Design review of the part built by this model. Coordinates are the model's own, in mm. A direction names the side the tool comes from. Coordinates: 2 decimals unless noted, no trailing zeros. Write each loop counter-clockwise with the first axis right and the second up, starting at its lowest first coordinate (ties: lowest second). Pieces come first, ordered by that corner, then holes.
Q1. For L1, parallel to Z at x = -5.5, y = 0; L2, parallel to Z at x = -6, y = 1.25; L3, parallel to Y at x = 3.75, z = 69.5, list the stretches that pass through material, from the lowest coordinate up.
Q2. The part is to be moulded in two halves that separate along Z. For faces 4 (the flat face through (13.97, 0, 50)), 5 (the cylindrical face through (-5.211, 0.112, 63.515)), 6 (the flat face through (0, 0, 101.6)), say which applies: released by +Z, released by -Z, zero draft, split by the parting line, or undercut.
Q3. Take a section at B-B, the plane z = 70.5. Write out the cut boundary in (x, y), plus the area to 3 significant figures.
Q4. Take a section at A-A, the plane y = 0. Write out the cut boundary in (x, z), plus the area to 3 significant figures.
Q5. For faces 1 (the cylindrical face through (6.348, 0.112, 53.952)), 2 (the cylindrical face through (-5.211, 0.112, 13.985)), 3 (the flat face through (0, 0, 0)), list the 3-axis set-ups (+Z, -Z, +X, -X, +Y, -Y) from which the entire face can be reached by the end or side of a thin tool; tool diameter is ignored.
Q6. Take a section at C-C, the plane x = -3.75. Write out the cut boundary in (y, z).
Q7. For pin 1 Ø6 at (y, z) = (-1, 83.5) entering from -X; pin 2 Ø2.5 at (x, y) = (4.5, -0.5) entering from +Z, all flat-tipped, find the tip position at first contact; note any pin that passes through.
from build123d import *

# Parameters (mm, degrees)
SKETCH1_W               = 27.94
SKETCH1_H               = 10.16
BOSS_EXTRUDE1_DEPTH     = 101.6
SKETCH3_R               = 2.5527
CUT_EXTRUDE2_DEPTH      = 96.148345755
CUT_EXTRUDE3_REACH      = 107.494
CUT_EXTRUDE3_END_RADIUS = 2.5527
SKETCH4_R               = 2.5527


with BuildPart() as part:
    # Sketch1 → Boss-Extrude1 (new body)
    with BuildSketch(Plane.XY):
        Rectangle(SKETCH1_W, SKETCH1_H)
    extrude(amount=BOSS_EXTRUDE1_DEPTH)

    # Sketch3 → Cut-Extrude2 (cut, through all)
    with BuildSketch(Plane(origin=(0, 0, 7.62), x_dir=(-1, 0, 0), z_dir=(0, 0, -1))):
        with Locations((-3.7973, 0)):
            Circle(SKETCH3_R)
    extrude(amount=-CUT_EXTRUDE2_DEPTH, mode=Mode.SUBTRACT)

    # Cut-Extrude3: up to this cylinder (the profile starts outside it)
    cut_extrude3_end = Plane(origin=(3.7973, 0, 49.5554), z_dir=(0, 0, -1)) * Cylinder(CUT_EXTRUDE3_END_RADIUS, 287.1334, mode=Mode.PRIVATE)
    # Sketch4 → Cut-Extrude3 (cut, up to the surface)
    with BuildSketch(Plane.ZY.offset(13.97), mode=Mode.PRIVATE) as cut_extrude3_sk1:
        with Locations((16.5354, 0)):
            Circle(SKETCH4_R)
    cut_extrude3_tool1 = extrude(cut_extrude3_sk1.sketch, amount=-CUT_EXTRUDE3_REACH, mode=Mode.PRIVATE) - cut_extrude3_end
    add(cut_extrude3_tool1.solids().sort_by_distance((-13.97, 0, 16.5354))[0], mode=Mode.SUBTRACT)
    # Sketch4 → Cut-Extrude3 (cut, up to the surface)
    with BuildSketch(Plane.ZY.offset(13.97), mode=Mode.PRIVATE) as cut_extrude3_sk2:
        with Locations((33.0454, 0)):
            Circle(SKETCH4_R)
    cut_extrude3_tool2 = extrude(cut_extrude3_sk2.sketch, amount=-CUT_EXTRUDE3_REACH, mode=Mode.PRIVATE) - cut_extrude3_end
    add(cut_extrude3_tool2.solids().sort_by_distance((-13.97, 0, 33.0454))[0], mode=Mode.SUBTRACT)
    # Sketch4 → Cut-Extrude3 (cut, up to the surface)
    with BuildSketch(Plane.ZY.offset(13.97), mode=Mode.PRIVATE) as cut_extrude3_sk3:
        with Locations((49.5554, 0)):
            Circle(SKETCH4_R)
    cut_extrude3_tool3 = extrude(cut_extrude3_sk3.sketch, amount=-CUT_EXTRUDE3_REACH, mode=Mode.PRIVATE) - cut_extrude3_end
    add(cut_extrude3_tool3.solids().sort_by_distance((-13.97, 0, 49.5554))[0], mode=Mode.SUBTRACT)
    # Sketch4 → Cut-Extrude3 (cut, up to the surface)
    with BuildSketch(Plane.ZY.offset(13.97), mode=Mode.PRIVATE) as cut_extrude3_sk4:
        with Locations((66.0654, 0)):
            Circle(SKETCH4_R)
    cut_extrude3_tool4 = extrude(cut_extrude3_sk4.sketch, amount=-CUT_EXTRUDE3_REACH, mode=Mode.PRIVATE) - cut_extrude3_end
    add(cut_extrude3_tool4.solids().sort_by_distance((-13.97, 0, 66.0654))[0], mode=Mode.SUBTRACT)
    # Sketch4 → Cut-Extrude3 (cut, up to the surface)
    with BuildSketch(Plane.ZY.offset(13.97), mode=Mode.PRIVATE) as cut_extrude3_sk5:
        with Locations((82.5754, 0)):
            Circle(SKETCH4_R)
    cut_extrude3_tool5 = extrude(cut_extrude3_sk5.sketch, amount=-CUT_EXTRUDE3_REACH, mode=Mode.PRIVATE) - cut_extrude3_end
    add(cut_extrude3_tool5.solids().sort_by_distance((-13.97, 0, 82.5754))[0], mode=Mode.SUBTRACT)


solid = part.part
Responses:
1. L1: z = 0 to 13.98, 19.09 to 30.49, 35.6 to 47, 52.11 to 63.51, 68.62 to 80.02, 85.13 to 101.6
1. L2: z = 0 to 14.31, 18.76 to 30.82, 35.27 to 47.33, 51.78 to 63.84, 68.29 to 80.35, 84.8 to 101.6
1. L3: y = -5.08 to -2.55, 2.55 to 5.08
2. face 4: zero draft
2. face 5: undercut
2. face 6: released by +Z
3. outline: (-13.97, -5.08) - (13.97, -5.08) - (13.97, 5.08) - (-13.97, 5.08) - close; hole circle Ø5.11 at (3.8, 0)
3. area: 263 mm2
4. outline: (-13.97, 0) - (13.97, 0) - (13.97, 101.6) - (6.35, 101.6) - (6.35, 7.62) - (1.24, 7.62) - (1.24, 13.98) - (-13.97, 13.98) - close; (-13.97, 19.09) - (1.24, 19.09) - (1.24, 30.49) - (-13.97, 30.49) - close; (-13.97, 35.6) - (1.24, 35.6) - (1.24, 47) - (-13.97, 47) - close; (-13.97, 52.11) - (1.24, 52.11) - (1.24, 63.51) - (-13.97, 63.51) - close; (-13.97, 68.62) - (1.24, 68.62) - (1.24, 80.02) - (-13.97, 80.02) - close; (-13.97, 85.13) - (1.24, 85.13) - (1.24, 101.6) - (-13.97, 101.6) - close
4. area: 1,970 mm2
5. face 1: +Z
5. face 2: -X
5. face 3: -Z, +X, -X, +Y, -Y
6. outline: (-5.08, 0) - (5.08, 0) - (5.08, 101.6) - (-5.08, 101.6) - close; hole circle Ø5.11 at (0, 16.54); hole circle Ø5.11 at (0, 33.05); hole circle Ø5.11 at (0, 49.56); hole circle Ø5.11 at (0, 66.07); hole circle Ø5.11 at (0, 82.58)
7. pin 1: stops at x = -13.97
7. pin 2: stops at z = 7.62
